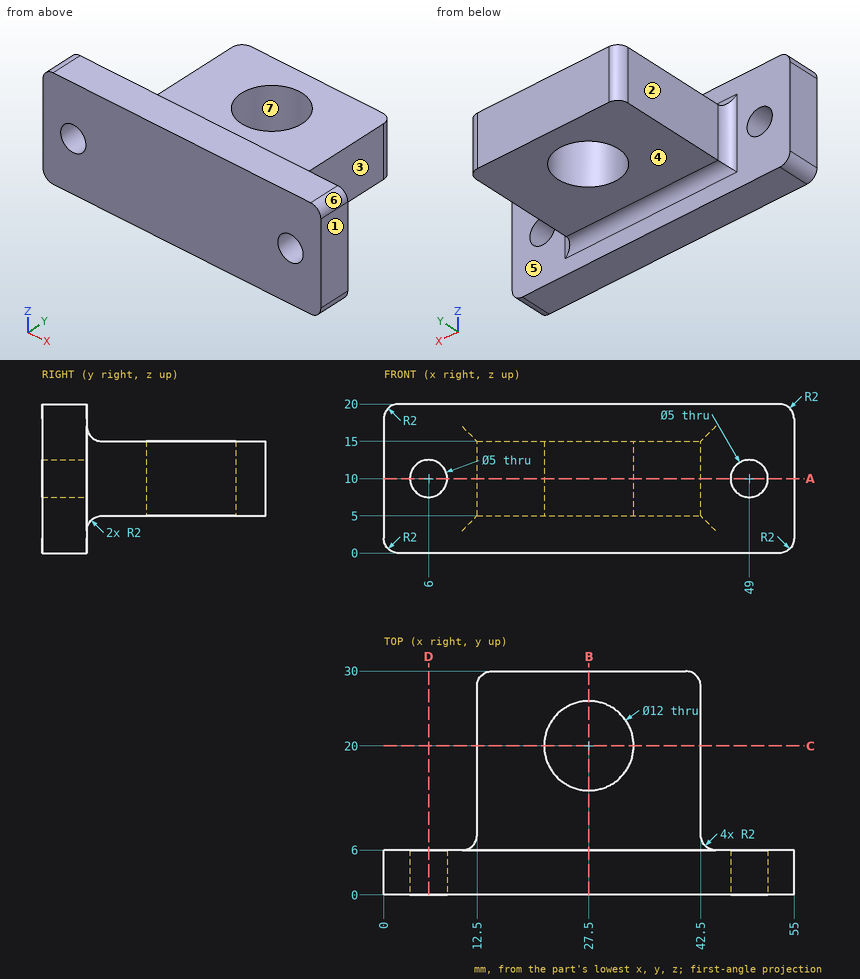
Study the drawing (mm; zero at the part's minimum x, y, z) and answer. A direction names the side the tool comes from. Coordinates: 2 decimals unless noted, no trailing zeros. Write each loop counter-clockwise with the first axis right and the second up, starting at its lowest first coordinate (ties: lowest second). Pieces come first, ordered by that corner, then holes. Notation, with made-up numbers: (24.5, 88.25) - (63.5, 88.25) arc R14 ccw to (63.5, 109.25) - close; hole circle Ø3 at (36.5, -18.75). An arc over 180 degrees is marked (long way). One line per question, with ' | ' between items.
1) The mould has two halves that part along X. Classify the marked faces 5, 6 and 7: +X half, -X half, draft (parallel to the pull), parting line (faces both ways), or undercut.
Checks:
face 5: draft | face 6: +X half | face 7: undercut
2) Find section B-B, the plane x = 27.5. Determine the outline of the cut face in (y, z), and give its area (3 significant figures).
Checks:
outline: (0, 0) - (6, 0) - (6, 3) arc R2 cw to (8, 5) - (14, 5) - (14, 15) - (8, 15) arc R2 cw to (6, 17) - (6, 20) - (0, 20) - close; (26, 5) - (30, 5) - (30, 15) - (26, 15) - close | area: 242 mm2
3) Find section C-C, the plane y = 20. Determine the outline of the cut face in (x, z), and give its area (3 significant figures).
Checks:
outline: (12.5, 5) - (21.5, 5) - (21.5, 15) - (12.5, 15) - close; (33.5, 5) - (42.5, 5) - (42.5, 15) - (33.5, 15) - close | area: 180 mm2
4) Consider probe 1 along Y at (x, z) = (27.5, 12.75); probe 2 along Y at (x, z) = (23, 1.75); probe 3 along X at (y, z) = (16, 9.25). Determine where each line is inside the solid, lowest interval first. Write a range as [from, to].
Checks:
probe 1: [0, 14], [26, 30] | probe 2: [0, 6] | probe 3: [12.5, 23.03], [31.97, 42.5]
5) Find section A-A, the plane z = 10. Determine the outline of the cut face in (x, y), and give its area (3 significant figures).
Checks:
outline: (0, 0) - (3.5, 0) - (3.5, 6) - (0, 6) - close; (8.5, 0) - (46.5, 0) - (46.5, 6) - (44.5, 6) arc R2 cw to (42.5, 8) - (42.5, 28) arc R2 ccw to (40.5, 30) - (14.5, 30) arc R2 ccw to (12.5, 28) - (12.5, 8) arc R2 cw to (10.5, 6) - (8.5, 6) - close; (51.5, 0) - (55, 0) - (55, 6) - (51.5, 6) - close; hole circle Ø12 at (27.5, 20) | area: 877 mm2
6) Flat-ended cylindrical pins translate along their axes: P1, Ø5, axis at y = 17, z = 9, coming from the -X side; P2, Ø6.5, axis at x = 49, z = 10, coming from the +Y side; P3, Ø11, axis at x = 23, y = 14.5, coming from the +Z side. Find the tip coordinate at first contact, or state that the pin passes through.
Checks:
P1: x = 12.5 | P2: y = 6 | P3: z = 15
7) For the marked faces 1, 2, 3 and 4, determine the directions among +Z, -Z, +X, -X, +Y, -Y from which every point of the face is accessible in a straight line to the end or side of a thin tool.
Checks:
face 1: +Z, -Z, +X, +Y, -Y | face 2: +Z, -Z, -X, +Y | face 3: +Z, -Z, +X, +Y | face 4: -Z, +X, -X, +Y
8) Find section D-D, the plane x = 6. Determine the outline of the cut face in (y, z), and give its area (3 significant figures).
Checks:
outline: (0, 0) - (6, 0) - (6, 7.5) - (0, 7.5) - close; (0, 12.5) - (6, 12.5) - (6, 20) - (0, 20) - close | area: 90.0 mm2
